Here's how the part is built. I have some questions about the finished solid (model axes, mm). Face numbers are marked on the shaded views. A direction names the side the tool comes from. Round coordinates to 2 decimals unless told otherwise and drop trailing zeros. Loops run counter-clockwise (first coordinate to the right, second up) from the corner with the lowest first, then second, coordinate; pieces in that order, holes last. Notation, with made-up numbers: M 41,23.25 L 55,23.25 A21 cw 55,54.25 Z; hole C 26,9.5 d8. An arc over 180 degrees is marked long. Use a Markdown table: item, result.
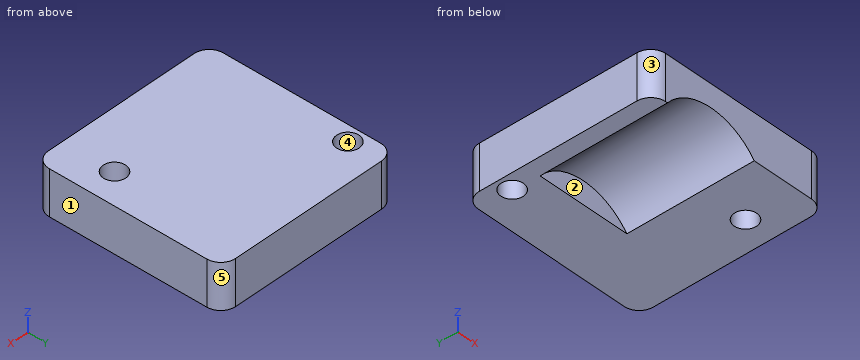
Autodesk Inventor part; units mm, degrees
ref_plane "YZ Plane" through (0, 0, 0) normal (1, 0, 0) x (0, 1, 0)
ref_plane "XZ Plane" through (0, 0, 0) normal (0, 1, 0) x (-1, 0, 0)
ref_plane "XY Plane" through (0, 0, 0) normal (0, 0, 1) x (1, 0, 0)
sketch "Sketch1" plane through (0, 0, 0) normal (0, 0, 1) x (1, 0, 0)
  circle A0 centre (21, 6.9652) radius 1.5 construction
  circle A1 centre (21, 6.9652) radius 1.5 construction
  line L0 (25, 0) -> (16.5, 0) construction
  line L1 (25, 0) -> (25, 55) construction
  line L2 (0, 55) -> (25, 55) construction
  line L3 (0, 0) -> (0, 55) construction
  line L4 (0.5, 0) -> (0, 0) construction
  line L5 (0.5, 17) -> (16.5, 17) construction
  circle A2 centre (16, 45) radius 7.5 construction
  line L6 (2, 25) -> (23, 25)
  line L7 (25, 23) -> (25, 2)
  line L8 (23, 0) -> (2, 0)
  line L9 (0, 2) -> (0, 23)
  circle A3 centre (21, 6.9652) radius 1.5
  arc A4 (2, 25) -> (0, 23) centre (2, 23) ccw
  arc A5 (0, 2) -> (2, 0) centre (2, 2) ccw
  arc A6 (23, 0) -> (25, 2) centre (23, 2) ccw
  arc A7 (25, 23) -> (23, 25) centre (23, 23) ccw
  circle A8 centre (2, 20.5) radius 1.5
  circle A9 centre (2, 20.5) radius 1.5
  line L10 (14.5, 12) -> (14.5, 6)
  line L11 (14.5, 6) -> (16.5, 6)
  line L12 (16.5, 6) -> (16.5, 0)
  line L13 (0.5, 0) -> (0.5, 6)
  line L14 (0.5, 6) -> (2.5, 6)
  line L15 (2.5, 6) -> (2.5, 12)
  line L16 (2.5, 12) -> (0.5, 12)
  line L17 (0.5, 12) -> (0.5, 17)
  line L18 (16.5, 17) -> (16.5, 12)
  line L19 (16.5, 12) -> (14.5, 12)
  point P0 (0, 25)
  dimension "d0" = 25
  dimension "d1" = 3
  dimension "d2" = 2
  dimension "d5" = 3
  dimension "d6" = 2
  dimension "d7" = 4.5
extrude "Extrusion1" add sketch "Sketch1" along normal blind 6
sketch "Sketch2" plane through (2, 0, 0) normal (0, -1, 0) x (1, 0, 0)
  circle A0 centre (6.5, -5) radius 8 construction
  circle A1 centre (6.5, -5) radius 8
  line L0 (21, 0) -> (0, 0)
  line L1 (0, 0) -> (0, 6)
  line L2 (21, 6) -> (0, 6)
  line L3 (21, 0) -> (21, 6)
  line L4 (12.745, 0) -> (0.255, 0)
  point P0 (-2, 0)
extrude "Extrusion2" cut sketch "Sketch2" against normal blind 17 contours L0 A1 picked at (4.8404, 0.4206)
properties part number "Hotend Lock 3"
Q1. We'd pull the mould along Y, two halves only. Please class the marked faces 3, 4 and 5: pulls with the +Y half, pulls with the -Y half, needs draft (parallel to the pull), parting line crosses it, or undercut.
Return value:
| item | result |
|---|---|
| face 3 | pulls with the -Y half |
| face 4 | undercut |
| face 5 | pulls with the +Y half |
Q2. I need wall thicknesses on line 1 (Y direction, x = 2, z = 1.5); line 2 (Y direction, x = 19.75, z = 2.75); line 3 (X direction, y = 11.25, z = 1). Which ranges of each line are inside material? Lowest first, please. Write a range as from..to.
Return value:
| item | result |
|---|---|
| line 1 | y = 0..19, 22..25 |
| line 2 | y = 0..6.14, 7.79..25 |
| line 3 | x = 0..3.21, 13.79..25 |
Q3. Imagine slicing it at B-B, the plane y = 20.5. Please give me the cut outline in (x, z).
Return value:
| item | result |
|---|---|
| outline | M 0,0 L 0.5,0 L 0.5,6 L 0,6 Z; M 3.5,0 L 25,0 L 25,6 L 3.5,6 Z |
Q4. Imagine slicing it at A-A, the plane x = 21. Please give me the cut outline in (y, z), then the cut area to 3 significant figures.
Return value:
| item | result |
|---|---|
| outline | M 0,0 L 5.47,0 L 5.47,6 L 0,6 Z; M 8.47,0 L 25,0 L 25,6 L 8.47,6 Z |
| area | 132 mm^2 |
Q5. For the marked faces 1 and 2, which set-ups out of +Z, -Z, +X, -X, +Y, -Y let a thin tool reach every point of the face, with its end or its side?
Return value:
| item | result |
|---|---|
| face 1 | +Z, -Z, +X, +Y, -Y |
| face 2 | -Z, -Y |
Q6. Imagine slicing it at C-C, the plane z = 1.5. Please give me the cut outline in (x, y).
Return value:
| item | result |
|---|---|
| outline | M 0,2 A2 ccw 2,0 L 3.84,0 L 3.84,17 L 13.16,17 L 13.16,0 L 23,0 A2 ccw 25,2 L 25,23 A2 ccw 23,25 L 2,25 A2 ccw 0,23 Z; hole C 2,20.5 d3; hole C 21,6.97 d3 |
Q7. Will this pin go through, and if not, where does the flat tip stop? P1, Ø0.9, axis at x = 7, z = 1.5, coming from the -Y side.
Return value:
| item | result |
|---|---|
| P1 | stops at y = 17 |
Q8. Imagine slicing it at D-D, the plane y = 3. Please give me the cut outline in (x, z) (3 decimals), then the cut area to 3 significant figures.
Return value:
| item | result |
|---|---|
| outline | M 0,0 L 2.255,0 A8 cw 14.745,0 L 25,0 L 25,6 L 0,6 Z |
| area | 124 mm^2 |
